Autodesk Inventor part; units mm, degrees
ref_plane "YZ Plane" through (0, 0, 0) normal (1, 0, 0) x (0, 1, 0)
ref_plane "XZ Plane" through (0, 0, 0) normal (0, 1, 0) x (-1, 0, 0)
ref_plane "XY Plane" through (0, 0, 0) normal (0, 0, 1) x (1, 0, 0)
sketch "Sketch1" plane through (0, 0, 0) normal (0, 1, 0) x (-1, 0, 0)
  line L0 (75, -49) -> (75, 49)
  line L1 (-75, 49) -> (-75, -49)
  line L2 (-75, -49) -> (75, 49) construction
  line L3 (75, -49) -> (-75, 49) construction
  line L4 (-40, -49) -> (-40, -19)
  line L5 (-40, -19) -> (40, -19)
  line L6 (40, -19) -> (40, -49)
  line L7 (-40, 49) -> (-40, 19)
  line L8 (-40, 19) -> (40, 19)
  line L9 (40, 19) -> (40, 49)
  line L10 (75, 49) -> (40, 49)
  line L11 (-40, 49) -> (-75, 49)
  line L12 (-75, -49) -> (-40, -49)
  line L13 (40, -49) -> (75, -49)
  point P0 (0, 0)
  dimension "d1" = 98
  dimension "d3" = 35
  dimension "d4" = 35
  dimension "d5" = 80
  dimension "d6" = 150
  dimension "d7" = 30
  dimension "d8" = 98
  dimension "d9" = 30
  dimension "d10" = 80
  dimension "d16" = 30
extrude "Main Body Extrusion" add sketch "Sketch1" along normal blind 6.5
sketch "Sketch2" plane through (-40, 0, 19) normal (0, 0, 1) x (1, 0, 0)
  line L0 (0, 0) -> (0, 6.5)
  line L1 (80, 0) -> (80, 6.5)
  line L2 (0, 6.5) -> (80, 6.5)
  line L3 (80, 6.5) -> (80, 2)
  line L4 (80, 2) -> (0, 2)
  line L5 (0, 2) -> (0, 6.5)
  point P0 (40, 0)
  dimension "d13" = 4.5
extrude "Center Cut" cut sketch "Sketch2" against normal up to next
sketch "Arc Sketch" plane through (75, 0, 49) normal (1, 0, 0) x (0, 0, -1)
  line L0 (49, 14.062) -> (49, -15.1255)
  line L1 (2, 11.8168) -> (2, -9.2171)
  line L2 (29, 10.0443) -> (29, -9.9261)
  line L3 (0, 0) -> (0, 6.5)
  line L4 (-6.6571, 2) -> (113.047, 2)
  line L5 (98, 0) -> (0, 0)
  line L6 (-13.629, 6) -> (113.047, 6)
  line L7 (15.5, 15.9527) -> (15.5, -15.1255)
  arc A0 (2, 6) -> (29, 6) centre (15.5, 26.7813) ccw
  line L8 (0, 6.5) -> (98, 6.5)
  line L9 (2, 6.5) -> (2, 6)
  line L10 (2, 6.5) -> (29, 6.5)
  line L11 (29, 6) -> (29, 6.5)
  arc A1 (69, 6) -> (96, 6) centre (82.5, 26.7813) ccw
  line L12 (96, 6.5) -> (96, 6)
  line L13 (96, 6.5) -> (69, 6.5)
  line L14 (69, 6) -> (69, 6.5)
  point P0 (49, 0)
  dimension "d17" = 2
  dimension "d18" = 2
  dimension "d19" = 4
  dimension "d20" = 27
  dimension "d21" = 13.5
  dimension "d24" = 15.5
extrude "Arc Cuts" cut sketch "Arc Sketch" against normal through all contours L2 L6 L7 L8 | L8 L12 L6 L14 | A0 L7 L6 | L6 A1 | L7 L6 L1 L8 | L7 A0 L6
sketch "Sketch4" plane through (0, 0, 0) normal (0, -1, 0) x (1, 0, 0)
  circle A0 centre (57.5, 33.5) radius 2
  line L0 (75, 49) -> (40, 49)
  line L1 (75, -49) -> (75, 49)
  line L2 (40, 49) -> (40, 19)
  line L3 (92.3487, 0) -> (-109.5218, 0)
  line L4 (0, -62.4236) -> (0, 64.0069)
  circle A1 centre (57.5, -33.5) radius 2
  circle A2 centre (-57.5, 33.5) radius 2
  circle A3 centre (-57.5, -33.5) radius 2
  line L5 (40, 19) -> (-40, 19)
  point P0 (0, 0)
  dimension "d25" = 4
  dimension "d26" = 15.5
  dimension "d27" = 17.5
  dimension "d28" = 35
  dimension "d41" = 14.5
  dimension "d42" = 17.5
extrude "Arc Holes Cut" cut sketch "Sketch4" against normal up to next contours A0 | A1 | A2 | A3
sketch "Sketch5" plane through (0, 6.5, 0) normal (0, 1, 0) x (1, 0, 0)
  line L0 (75, 47) -> (75, 49)
  line L1 (40, 49) -> (75, 49)
  line L2 (75, 47) -> (40, 47)
  line L3 (40, 47) -> (40, 49)
  line L4 (40, 49) -> (75, 49)
  line L5 (75, 49) -> (75, 47)
  line L6 (88.7308, 0) -> (-106.3834, 0)
  line L7 (0, 126.6929) -> (0, -73.8866)
  line L8 (75, -47) -> (75, -49)
  line L9 (40, -49) -> (75, -49)
  line L10 (75, -47) -> (40, -47)
  line L11 (40, -47) -> (40, -49)
  line L12 (-75, 47) -> (-75, 49)
  line L13 (-40, 49) -> (-75, 49)
  line L14 (-75, 47) -> (-40, 47)
  line L15 (-40, 47) -> (-40, 49)
  line L16 (-75, -47) -> (-40, -47)
  line L17 (-40, -49) -> (-75, -49)
  line L18 (-75, -47) -> (-75, -49)
  line L19 (-40, -47) -> (-40, -49)
  point P0 (0, 0)
extrude "Side Extrusions" add sketch "Sketch5" along normal blind 10
sketch "Side Holes Sketch" plane through (-40, 0, -49) normal (0, 0, -1) x (-1, 0, 0)
  circle A0 centre (-106.25, 11.25) radius 2
  line L0 (-115, 6) -> (-80, 6)
  line L1 (-80, 0) -> (-115, 0)
  line L2 (-115, 16.5) -> (-80, 16.5)
  line L3 (-97.5, 0) -> (-97.5, 22.5291)
  line L4 (-115, 0) -> (-115, 16.5)
  circle A1 centre (-88.75, 11.25) radius 2
  line L5 (-40, 14.9188) -> (-40, -21.0119)
  circle A2 centre (26.25, 11.25) radius 2
  circle A3 centre (8.75, 11.25) radius 2
  point P0 (-40, 0)
  dimension "d33" = 6
  dimension "d34" = 10.5
  dimension "d35" = 5.25
  dimension "d36" = 5.25
  dimension "d37" = 35
  dimension "d38" = 8.75
  dimension "d56" = 4
extrude "Side Holes Cut" cut sketch "Side Holes Sketch" against normal through all contours A0 | A1 | A2 | A3
sketch "Ramp Width Sketch" plane through (-75, 0, -49) normal (-1, 0, 0) x (0, 0, 1)
  line L0 (96, 6) -> (96, 16.5)
  line L1 (2, 0) -> (96, 0)
  line L2 (96, 0) -> (96, 8)
  line L3 (96, 8) -> (2, 8)
  line L4 (2, 8) -> (2, 0)
  point P0 (49, 0)
  dimension "d43" = 8
  dimension "d44" = 94
extrude "Ramp Width Extrusion" add sketch "Ramp Width Sketch" along normal blind 21.9798
sketch "Ramp Cut Sketch" plane through (-75, 0, 47) normal (0, 0, 1) x (1, 0, 0)
  line L0 (0, 16.5) -> (0, 8)
  line L1 (-21.9798, 0) -> (-21.9798, 8)
  line L2 (0, 8) -> (-21.9798, 0)
  line L3 (0, 8) -> (-21.9798, 8)
  line L4 (-21.9798, 8) -> (0, 8)
  point P0 (75, 0)
extrude "Ramp Cut" cut sketch "Ramp Cut Sketch" against normal through all
sketch "Sketch12" plane through (0, 0, 0) normal (0, -1, 0) x (1, 0, 0)
  line L0 (74.2886, 0) -> (75, 0)
  line L1 (75, 49) -> (40, 49)
  line L2 (40, -49) -> (75, -49)
  line L3 (75, -49) -> (75, 49)
  line L4 (75, 3.5) -> (78.5, 3.5)
  line L5 (78.5, -3.5) -> (75, -3.5)
  line L6 (75, -3.5) -> (75, 3.5)
  arc A0 (78.5, -3.5) -> (78.5, 3.5) centre (78.5, 0) ccw
  point P0 (0, 0)
  dimension "d49" = 49
  dimension "d50" = 49
  dimension "d51" = 3.5
  dimension "d52" = 3.5
extrude "Extrusion9" add sketch "Sketch12" against normal blind 6.5
sketch "Sketch13" plane through (0, 6.5, 0) normal (0, 1, 0) x (1, 0, 0)
  arc A0 (78.5, -3.5) -> (78.5, 3.5) centre (78.5, 0) ccw
  circle A1 centre (78.5, 0) radius 1
  point P0 (0, 0)
  dimension "d57" = 2
extrude "Extrusion10" cut sketch "Sketch13" against normal through all
properties part number "TapeMeasureBracketBottom"
Model file for the job. Use its own axes, mm. A direction names the side the tool comes from. Coordinates: 2 decimals unless noted, no trailing zeros. Order: outer loops, then holes, each group sorted by start corner. A loop starts at its lowest first (then second) coordinate and runs counter-clockwise, first axis right, second up. Notation, with made-up numbers: M -24,11.5 L 35,11.5 A28 cw 35,44.5 Z; hole C 42,82.25 d6. An arc over 180 degrees is marked long. Answer as CSV lines item,"result".
(1) Band-saw the part on B-B, the plane z = 33.5. List the corners of the cut face in (x, y), then the cut area to 3 significant figures.
Geometry says:
outline,"M -96.98,0 L -59.5,0 L -59.5,2 L -75,2 L -75,8 Z; M -55.5,0 L -40,0 L -40,2 L -55.5,2 Z; M 40,0 L 55.5,0 L 55.5,2 L 40,2 Z; M 59.5,0 L 75,0 L 75,2 L 59.5,2 Z"
area,"212 mm2"
(2) Wall check: line 1 along Z through (x, y) = (-57.5, 0.8); line 2 along Y through (x, z) = (66.25, 47.9); line 3 along Z through (x, y) = (41, 12.25). Give the ranges that are in metal, low to high.
Geometry says:
line 1,"z = -49 to -35.5, -31.5 to 31.5, 35.5 to 49"
line 2,"y = 0 to 9.25, 13.25 to 16.5"
line 3,"z = -49 to -47, 47 to 49"
(3) Flat gauge pins, fed straight in: pin 1 (8 mm diameter, centred on x = 32, y = 4.5, fed in from -Z); pin 2 (17.5 mm diameter, centred on x = -51.5, z = 8.5, fed in from +Y); pin 3 (2.5 mm diameter, centred on x = 48.75, y = 11.25, fed in from -Z); pin 4 (5 mm diameter, centred on y = 10, z = -36.5, fed in from +X). Where does each tip first touch, or does it go through?
Geometry says:
pin 1,"stops at z = -19"
pin 2,"stops at y = 6.5"
pin 3,"passes through"
pin 4,"stops at x = -75"
(4) Band-saw the part on A-A, the plane x = -66.25. List the corners of the cut face in (y, z), then the cut area to 3 significant figures.
Geometry says:
outline,"M 0,-49 L 9.25,-49 L 9.25,-47 L 6,-47 A24.78 cw 6,-20 L 6.5,-20 L 6.5,20 L 6,20 A24.78 cw 6,47 L 9.25,47 L 9.25,49 L 0,49 Z; M 13.25,-49 L 16.5,-49 L 16.5,-47 L 13.25,-47 Z; M 13.25,47 L 16.5,47 L 16.5,49 L 13.25,49 Z"
area,"488 mm2"
(5) Band-saw the part on C-C, the plane y = 11.25. State how many separate pieces and enclosed holes the cut face has, then the cut area to 3 significant figures.
Geometry says:
separate pieces,"12"
enclosed holes,"0"
area,"216 mm2"
(6) Band-saw the part on D-D, the plane z = -9. List the corners of the cut face in (x, y), then the cut area to 3 significant figures.
Geometry says:
outline,"M -96.98,0 L 75,0 L 75,6.5 L 40,6.5 L 40,2 L -40,2 L -40,6.5 L -75,6.5 L -75,8 Z"
area,"703 mm2"
(7) Pull direction X, two halves, no side cores. Call faces 1 (the flat face through (-57, 6.5, 0)), 2 (the cylindrical face through (-56.577, 1.026, -35.274)), 3 (the flat face through (75, 3, 25)): +X half, -X half, draft (parallel to the pull), parting line (faces both ways), or undercut.
Geometry says:
face 1,"draft"
face 2,"undercut"
face 3,"+X half"
(8) 3-axis set-ups, long thin cutter, end or side, ignore diameter. For faces 4 (the flat face through (-57, 11, -47)), 5 (the flat face through (-81, 2, -47)), 6 (the flat face through (1, 2, 0)): which of +Z, -Z, +X, -X, +Y, -Y reach the whole face in a straight line?
Geometry says:
face 4,"+X, +Y"
face 5,"-Z, -X, +Y, -Y"
face 6,"+Z, -Z, +Y"
